from build123d import *

# Parameters (mm, degrees)
F1_DEPTH = 15
F2_R     = 3
F3_DEPTH = 25
F4_R     = 2.99999


# Not quite as in the source:
# - a fillet or chamfer is up to 0.001 mm smaller than in the source, because OpenCascade refuses the exact size


with BuildPart() as f1:
    # F0 (on Top) → F1 (new body)
    with BuildSketch(Plane.XY):
        Polygon((-6, 0), (0, 0), (0, 40), (-20, 40), (-31.8061554718, 17.9633329885), (-6, 17.9633329885), align=None)
    extrude(amount=F1_DEPTH)

    # F2 (on face) → F3 (cut)
    with BuildSketch(Plane.XY.offset(15)):
        with Locations((-6, 25)):
            Circle(F2_R)
    extrude(amount=-F3_DEPTH, mode=Mode.SUBTRACT)

    # F4 (radius 3 in the source; OpenCascade refuses exactly that, so slightly less here)
    f4_edges = [f1.edges().sort_by_distance(p)[0] for p in [
        (0, 20, 15),
        (-6, 8.981666, 15),
        (-18.903078, 17.963333, 15),
        (-25.903078, 28.981666, 15),
        (-10, 40, 15),
        (0, 40, 7.5),
        (-3, 0, 15),
        (0, 0, 7.5),
        (0, 20, 0),
        (-18.903078, 17.963333, 0),
        (-31.806155, 17.963333, 7.5),
        (-6, 0, 7.5),
    ]]
    fillet(f4_edges, radius=F4_R)


solid = f1.part
Input: part model. Units: mm. Frame: model coordinates. A direction names the side the tool comes from. Coordinates: 2 decimals unless noted, no trailing zeros. Loops run counter-clockwise (first coordinate to the right, second up) from the corner with the lowest first, then second, coordinate; pieces in that order, holes last.
Q1. Draft query along Y for faces 1 (the face through (-24.654, 31.313, 5.916)), 2 (the face through (-13, 28, 15)), 3 (the face through (-17, 17.963, 7)), 4 (the face through (-3.23, 23.85, 7.6)). Return one class per face: +Y half, -Y half, draft (parallel to the pull), parting line (faces both ways), or undercut.
Q2. Cut plane A-A (x = -6.75). Output: boundary loops of the cut face in (y, z).
Q3. Set-up query: faces 5 (the face through (-5.14, 11.86, 14.1)), 6 (the face through (-17.731, 18.865, 0.855)), 7 (the face through (-29.35, 19.39, 6.08)). Return all of +Z, -Z, +X, -X, +Y, -Y with unobstructed straight access to the full face (end or side cutting, diameter ignored); none if empty.
Q4. Cut plane C-C (x = -17.25). Output: boundary loops of the cut face in (y, z).
Q5. Material intervals for line 1 (Y direction, x = -4, z = 3.25); line 2 (Y direction, x = -18.25, z = 8.5); line 3 (X direction, y = 26, z = 1.75), sorted ascending.
Q6. Cut plane D-D (x = -2). Output: boundary loops of the cut face in (y, z).
Q7. Contact query for flat-ended pins moving along their axis: pin 1 (3 mm diameter, centred on x = -24.5, y = 32.5, fed in from +Z); pin 2 (5 mm diameter, centred on x = -6, y = 25, fed in from +Z). Output: stop coordinate, or through.
Working result:
1. face 1: +Y half
1. face 2: draft
1. face 3: -Y half
1. face 4: undercut
2. outline: (17.96, 3) arc R3 ccw to (20.96, 0) - (22.1, 0) - (22.1, 15) - (20.96, 15) arc R3 ccw to (17.96, 12) - close; (27.9, 0) - (40, 0) - (40, 12) arc R3 ccw to (37, 15) - (27.9, 15) - close
3. face 5: +Z, -X, -Y
3. face 6: -Z, -X, -Y
3. face 7: +Z, -Z, -X
4. outline: (17.96, 3) arc R3 ccw to (20.96, 0) - (40, 0) - (40, 12) arc R3 ccw to (37, 15) - (20.96, 15) arc R3 ccw to (17.96, 12) - close
5. line 1: y = 0.17 to 22.76, 27.24 to 40
5. line 2: y = 17.96 to 40
5. line 3: x = -27.5 to -8.83, -3.17 to -0.27
6. outline: (0.17, 0.17) - (39.83, 0.17) - (39.83, 12) arc R2.83 ccw to (37, 14.83) - (3, 14.83) arc R2.83 ccw to (0.17, 12) - close
7. pin 1: stops at z = 14.3
7. pin 2: passes through
